Design review of the part shown in the three views and the two pictorial views. Dimensions are in mm from the part's minimum x, y and z. A direction names the side the tool comes from. Give positions to 0.01 mm unless a question says otherwise; leave off trailing zeros. Loops run counter-clockwise (first coordinate to the right, second up) from the corner with the lowest first, then second, coordinate; pieces in that order, holes last. Notation, with made-up numbers: (0, -15.5) - (30, -15.5) arc R17 cw to (30, 14.5) - close; hole circle Ø11 at (85.5, 12.25). An arc over 180 degrees is marked (long way). Put each result on its own line as item: value. Start each with the question number.
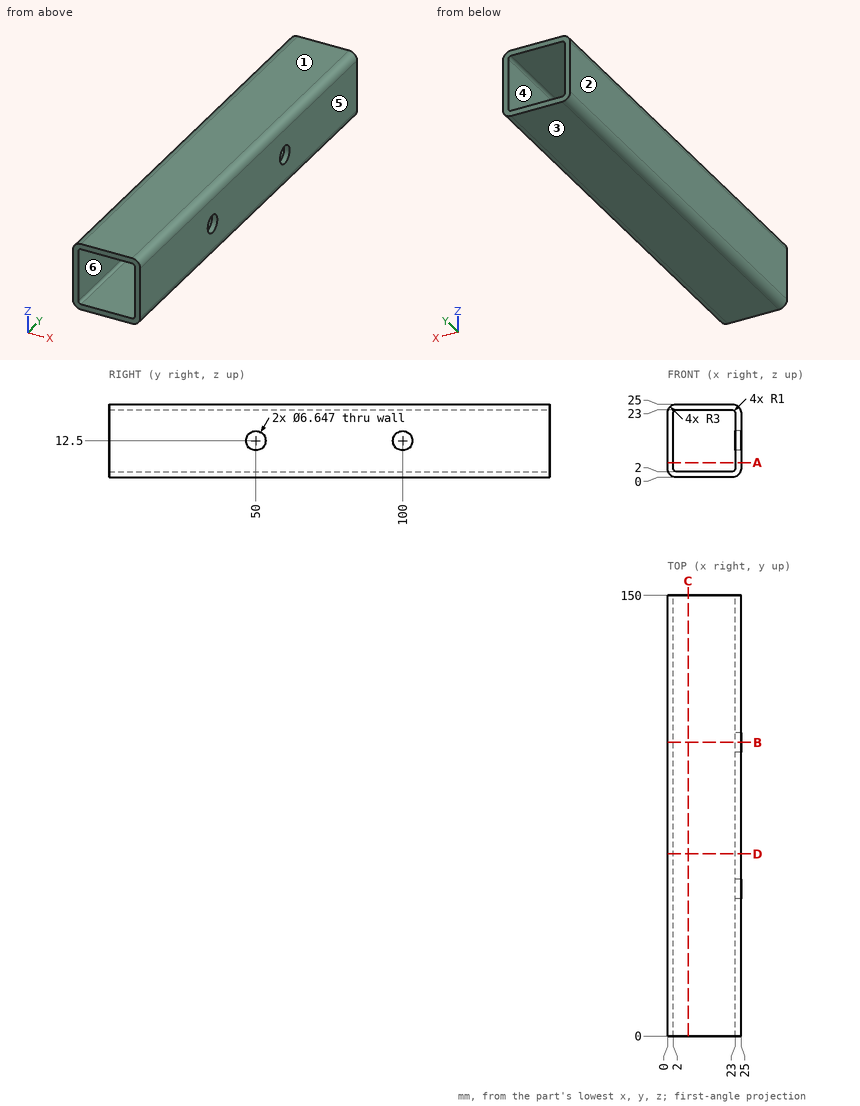
1) Machinability: for the marked faces 5 and 6, which of the approach directions +Z, -Z, +X, -X, +Y, -Y give a long, thin tool a straight path to every point of the face, cutting with its end or side? Answer none if there is none.
2) Take a section at A-A on z = 5. State the section outline as (x, y) points.
3) Take a section at B-B on y = 100. State the section outline as (x, z) points.
4) Mouldability with a two-part tool opening along Z and no side actions: class the marked faces 1, 2, 3 and 4 as released by +Z, released by -Z, zero draft, split by the parting line, or undercut.
5) Take a section at C-C on x = 7. State the section outline as (y, z) points, and give its area (3 significant figures).
6) Wall thickness on probe 1 along Y at (x, z) = (23.8, 12.5); probe 2 along X at (y, z) = (142, 17.25): over which ranges is each line inside the solid? List them lowest first.
7) Take a section at D-D on y = 62. State the section outline as (x, z) points, and give its area (3 significant figures).
Answers follow:
1. face 5: +Z, -Z, +X, +Y, -Y
1. face 6: +Y, -Y
2. outline: (0, 0) - (2, 0) - (2, 150) - (0, 150) - close; (23, 0) - (25, 0) - (25, 150) - (23, 150) - close
3. outline: (0, 3) arc R3 ccw to (3, 0) - (22, 0) arc R3 ccw to (25, 3) - (25, 9.18) - (23, 9.18) - (23, 3) arc R1 cw to (22, 2) - (3, 2) arc R1 cw to (2, 3) - (2, 22) arc R1 cw to (3, 23) - (22, 23) arc R1 cw to (23, 22) - (23, 15.82) - (25, 15.82) - (25, 22) arc R3 ccw to (22, 25) - (3, 25) arc R3 ccw to (0, 22) - close
4. face 1: released by +Z
4. face 2: zero draft
4. face 3: released by -Z
4. face 4: undercut
5. outline: (0, 0) - (150, 0) - (150, 2) - (0, 2) - close; (0, 23) - (150, 23) - (150, 25) - (0, 25) - close
5. area: 600 mm2
6. probe 1: 0 to 46.68, 53.32 to 96.68, 103.32 to 150
6. probe 2: 0 to 2, 23 to 25
7. outline: (0, 3) arc R3 ccw to (3, 0) - (22, 0) arc R3 ccw to (25, 3) - (25, 22) arc R3 ccw to (22, 25) - (3, 25) arc R3 ccw to (0, 22) - close; hole (2, 3) arc R1 ccw to (3, 2) - (22, 2) arc R1 ccw to (23, 3) - (23, 22) arc R1 ccw to (22, 23) - (3, 23) arc R1 ccw to (2, 22) - close
7. area: 177 mm2
